Read the model definition and answer for the solid it produces. Units are mm, in the model's axes. Coordinates: 2 decimals unless noted, no trailing zeros. Loops run counter-clockwise (first coordinate to the right, second up) from the corner with the lowest first, then second, coordinate; pieces in that order, holes last. Notation, with made-up numbers: (62, 11.5) -> (70, 11.5) arc R8 cw to (70, 20.5) -> close; hole circle Ø4 at (-14.75, 61). An arc over 180 degrees is marked (long way). Answer as a JSON object with one key per item and string values. Group by question number.
Q1. Each of these flat-tipped pins is pushed along its axis until it touches: P1, Ø1, axis at x = 10.5, z = 2, coming from the +Y side; P2, Ø4.5, axis at x = 0, y = 20, coming from the +Z side. Where does it stop, or does it pass through?
Q2. The part is cut by section A-A on x = 0. Write down the section's boundary in (y, z), and give its area (3 significant figures).
Q3. Straight lines are drawn through the part: line 1 along Y through (x, z) = (0, 1.4); line 2 along Y through (x, z) = (-1, 0.7); line 3 along X through (y, z) = (20.5, 1.35). For each, find the intervals that lie inside material, in ascending order. Write a range as [from, to].
Q4. Determine the mould class of faces 1 (the cylindrical face through (0.26, 21.983, 1.493)), 2 (the cylindrical face through (-0.2, -25, 1.5)), 3 (the flat face through (15, -0.2, 1.5)) for opening direction Y: released by +Y, released by -Y, zero draft, split by the parting line, or undercut.
from build123d import *

# Parameters (mm, degrees)
F1_DEPTH = 3
F3_D     = 4
F4_R     = 1


# Not quite as in the source:
# - ends of sketch curves that miss each other by under 0.0002 mm in the source are joined


with BuildPart() as f1:
    # F0 (on Top) → F1 (new body)
    with BuildSketch(Plane.XY):
        with BuildLine():
            Line((15, -15), (15, 15.0000007931))
            ThreePointArc((15, 15.0000007931), (14.4074542357, 17.7922023165), (12.7319587629, 20.1030927835))
            ThreePointArc((12.7319587629, 20.1030927835), (0, 25), (-12.7319587629, 20.1030927835))
            ThreePointArc((-12.7319587629, 20.1030927835), (-14.4074543968, 17.7922019541), (-15, 15))
            Line((-15, 15), (-15, -15.0000007931))
            ThreePointArc((-15, -15.0000007931), (-14.4074543968, -17.7922019541), (-12.7319587629, -20.1030927835))
            ThreePointArc((-12.7319587629, -20.1030927835), (0, -25), (12.7319587629, -20.1030927835))
            ThreePointArc((12.7319587629, -20.1030927835), (14.4074542357, -17.7922023165), (15, -15))
        make_face()
    extrude(amount=F1_DEPTH)

    # F3 (through all)
    with Locations(Plane.XY.offset(3)):
        with Locations((0, 20)):
            Hole(F3_D / 2)

    # F4
    f4_edges = [f1.edges().sort_by_distance(p)[0] for p in [
        (14.407454, -17.792202, 3),
        (0, -25, 3),
        (15, 0, 3),
        (-14.407454, -17.792202, 3),
        (14.407454, 17.792202, 3),
        (-15, 0, 3),
        (0, 25, 3),
        (-14.407454, 17.792202, 3),
        (-2, 20, 3),
        (14.407454, -17.792202, 0),
        (0, -25, 0),
        (15, 0, 0),
        (-14.407454, -17.792202, 0),
        (14.407454, 17.792202, 0),
        (-15, 0, 0),
        (0, 25, 0),
        (-14.407454, 17.792202, 0),
        (-2, 20, 0),
    ]]
    fillet(f4_edges, radius=F4_R)


solid = f1.part
Final values:
{
 "1": {"P1": "stops at y = 22.16", "P2": "stops at z = 2.66"},
 "2": {"outline": "(-25, 1) arc R1 ccw to (-24, 0) -> (17, 0) arc R1 ccw to (18, 1) -> (18, 2) arc R1 ccw to (17, 3) -> (-24, 3) arc R1 ccw to (-25, 2) -> close; (22, 1) arc R1 ccw to (23, 0) -> (24, 0) arc R1 ccw to (25, 1) -> (25, 2) arc R1 ccw to (24, 3) -> (23, 3) arc R1 ccw to (22, 2) -> close", "area": "136 mm2"},
 "3": {"line 1": "y = [-25, 18], [22, 25]", "line 2": "y = [-24.93, 18.21], [21.79, 24.93]", "line 3": "x = [-12.28, -1.94], [1.94, 12.28]"},
 "4": {"face 1": "undercut", "face 2": "released by -Y", "face 3": "zero draft"}
}
